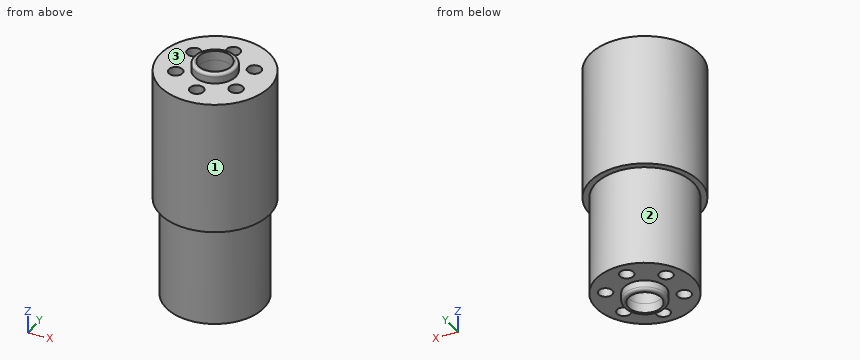
```python
from build123d import *

# Parameters (mm, degrees)
SKETCH1_R           = 25.4
BOSS_EXTRUDE2_DEPTH = 108.458
SKETCH6_R           = 7.62
SKETCH6_R_2         = 3.175
CUT_EXTRUDE1_DEPTH  = 108.458
SKETCH7_R           = 25.4
SKETCH7_R_2         = 22.606
CUT_EXTRUDE2_DEPTH  = 46.482
SKETCH8_R           = 9.652
SKETCH8_R_2         = 7.62
BOSS_EXTRUDE7_DEPTH = 4.4577
BOSS_EXTRUDE8_START = 4.4577
SKETCH9_R           = 9.652
SKETCH9_R_2         = 7.62
BOSS_EXTRUDE8_DEPTH = 4.4577
FILLET1_R           = 1.27


with BuildPart() as part:
    # Sketch1 → Boss-Extrude2 (new body)
    with BuildSketch(Plane.XY):
        Circle(SKETCH1_R)
    extrude(amount=BOSS_EXTRUDE2_DEPTH)

    # Sketch6 → Cut-Extrude1 (cut)
    with BuildSketch(Plane(origin=(0, 0, 0), x_dir=(-1, 0, 0), z_dir=(0, 0, -1))):
        Circle(SKETCH6_R)
        with Locations((-13.858138511, 8.001)):
            Circle(SKETCH6_R_2)
        with Locations((0, 16.002)):
            Circle(SKETCH6_R_2)
        with Locations((13.858138511, 8.001)):
            Circle(SKETCH6_R_2)
        with Locations((13.858138511, -8.001)):
            Circle(SKETCH6_R_2)
        with Locations((0, -16.002)):
            Circle(SKETCH6_R_2)
        with Locations((-13.858138511, -8.001)):
            Circle(SKETCH6_R_2)
    extrude(amount=-CUT_EXTRUDE1_DEPTH, mode=Mode.SUBTRACT)

    # Sketch7 → Cut-Extrude2 (cut)
    with BuildSketch(Plane(origin=(0, 0, 0), x_dir=(-1, 0, 0), z_dir=(0, 0, -1))):
        Circle(SKETCH7_R)
        Circle(SKETCH7_R_2, mode=Mode.SUBTRACT)
    extrude(amount=-CUT_EXTRUDE2_DEPTH, mode=Mode.SUBTRACT)

    # Sketch8 → Boss-Extrude7 (add)
    with BuildSketch(Plane.XY.offset(108.458)):
        Circle(SKETCH8_R)
        with Locations(Location((0, 0, 0), (0, 0, 180))):
            Circle(SKETCH8_R_2, mode=Mode.SUBTRACT)
    extrude(amount=BOSS_EXTRUDE7_DEPTH)

    # Sketch9 → Boss-Extrude8 (add)
    with BuildSketch(Plane(origin=(0, 0, 0), x_dir=(-1, 0, 0), z_dir=(0, 0, -1)).offset(BOSS_EXTRUDE8_START)):
        with Locations(Location((0, 0, 0), (0, 0, 180))):
            Circle(SKETCH9_R)
        Circle(SKETCH9_R_2, mode=Mode.SUBTRACT)
    extrude(amount=-BOSS_EXTRUDE8_DEPTH)

    # Fillet1
    fillet1_edges = [part.edges().sort_by_distance(p)[0] for p in [
        (-9.652, 0, 112.9157),
        (-9.652, 0, -4.4577),
    ]]
    fillet(fillet1_edges, radius=FILLET1_R)


solid = part.part
```
Source: CAD feature listing. Evaluate the final solid. Frame: model axes, mm. Face numbers are marked on the shaded views. A direction names the side the tool comes from. Give positions to 0.01 mm unless a question says otherwise; leave off trailing zeros. Write each loop counter-clockwise with the first axis right and the second up, starting at its lowest first coordinate (ties: lowest second). Pieces come first, ordered by that corner, then holes.
1. Material intervals for line 1 along Y through (x, z) = (0, 86); line 2 along Y through (x, z) = (0, 28); line 3 along X through (y, z) = (-8, 71), sorted ascending.
2. Access query for the marked faces 1, 2 and 3. Directions: +Z, -Z, +X, -X, +Y, -Y. A direction counts if a zero-diameter tool reaches every point of the face in a straight line with its end or side. Return the directions, or none.
3. Section query A-A (y = 0). Return the cut outline in (x, z), then the cut area to 3 significant figures.
4. Section query D-D (x = -12). Return the cut outline in (y, z).
5. Section query C-C (z = 25.5). Return the cut outline in (x, y) (3 decimals), then the cut area to 3 significant figures.
6. Section query B-B (x = 0). Count the separate pieces of the cut face and the enclosed holes in it, then the cut area to 3 significant figures.
7. First-contact query: pin 1 (6 mm diameter, centred on x = 5, z = 45.5, fed in from -Y); pin 2 (8.5 mm diameter, centred on x = 0, y = -16.002, fed in from -Z); pin 3 (5 mm diameter, centred on x = -2, z = 96, fed in from +Y). Flat tips, straight axial feed; report the tip coordinate or a pass-through.
Output values:
1. line 1: y = -25.4 to -19.18, -12.83 to -7.62, 7.62 to 12.83, 19.18 to 25.4
1. line 2: y = -22.61 to -19.18, -12.83 to -7.62, 7.62 to 12.83, 19.18 to 22.61
1. line 3: x = -24.11 to -17.03, -10.68 to 10.68, 17.03 to 24.11
2. face 1: +Z, -Z
2. face 2: -Z
2. face 3: +Z
3. outline: (-25.4, 46.48) - (-22.61, 46.48) - (-22.61, 0) - (-9.65, 0) - (-9.65, -3.19) arc R1.27 ccw to (-8.38, -4.46) - (-7.62, -4.46) - (-7.62, 112.92) - (-8.38, 112.92) arc R1.27 ccw to (-9.65, 111.65) - (-9.65, 108.46) - (-25.4, 108.46) - close; (7.62, -4.46) - (8.38, -4.46) arc R1.27 ccw to (9.65, -3.19) - (9.65, 0) - (22.61, 0) - (22.61, 46.48) - (25.4, 46.48) - (25.4, 108.46) - (9.65, 108.46) - (9.65, 111.65) arc R1.27 ccw to (8.38, 112.92) - (7.62, 112.92) - close
3. area: 3,630 mm2
4. outline: (-22.39, 46.48) - (-19.16, 46.48) - (-19.16, 0) - (-10.58, 0) - (-10.58, 108.46) - (-22.39, 108.46) - close; (-5.43, 0) - (5.43, 0) - (5.43, 108.46) - (-5.43, 108.46) - close; (10.58, 0) - (19.16, 0) - (19.16, 46.48) - (22.39, 46.48) - (22.39, 108.46) - (10.58, 108.46) - close
5. outline: circle Ø45.212 at (0, 0); hole circle Ø6.35 at (-13.858, -8.001); hole circle Ø6.35 at (-13.858, 8.001); hole circle Ø15.24 at (0, 0); hole circle Ø6.35 at (0, -16.002); hole circle Ø6.35 at (0, 16.002); hole circle Ø6.35 at (13.858, -8.001); hole circle Ø6.35 at (13.858, 8.001)
5. area: 1,230 mm2
6. separate pieces: 4
6. enclosed holes: 0
6. area: 2,250 mm2
7. pin 1: stops at y = -25.31
7. pin 2: stops at z = 0
7. pin 3: stops at y = 25.4
